For this review, take the finished solid that the model builds, in its own axes (mm). Face numbers are marked on the shaded views. A direction names the side the tool comes from. Coordinates: 2 decimals unless noted, no trailing zeros. Order: outer loops, then holes, each group sorted by start corner. A loop starts at its lowest first (then second) coordinate and runs counter-clockwise, first axis right, second up. Notation, with made-up numbers: (9, 85) - (14, 85) arc R25 cw to (14, 113) - close; hole circle Ø7 at (-1.5, 88.25). An arc over 180 degrees is marked (long way). One line per item, written item: value. Start each with the question number.
(1) Clearance check with flat-ended pins moving along their axes: pin 1 (2 mm diameter, centred on y = 21, z = 2.5, fed in from -X); pin 2 (2 mm diameter, centred on y = 14, z = 2, fed in from -X); pin 3 (1.6 mm diameter, centred on x = 34.5, z = 2.5, fed in from -Y). State where each tip first meets the part, or that it passes through.
(2) Consider section C-C on y = 10. Write out the cut boundary in (x, z), then the cut area to 3 significant figures.
(3) To check wall thickness, follow line 1 along X through (y, z) = (6.5, 3.7); line 2 along X through (y, z) = (4.25, 3.25); line 3 along Y through (x, z) = (44.5, 3.1). State the ranges of each line that lie inside material, in increasing order.
(4) Consider section D-D on y = 16.45. Write out the cut boundary in (x, z).
(5) Consider section A-A on x = 44.5. Write out the cut boundary in (y, z).
(6) For the marked faces 1, 2 and 3, list the 3-axis set-ups (+Z, -Z, +X, -X, +Y, -Y) from which the entire face can be reached by the end or side of a thin tool; tool diameter is ignored.
(7) Mouldability with a two-part tool opening along X and no side actions: class the marked faces 4, 5, 6 and 7 as released by +X, released by -X, zero draft, split by the parting line, or undercut.
(8) Consider section B-B on z = 0.75. Write out the cut boundary in (x, y), then the cut area to 3 significant figures.
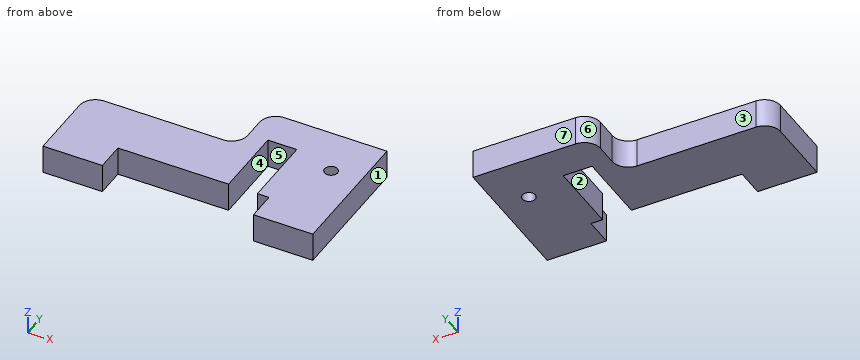
```python
from build123d import *

# Parameters (mm, degrees)
MODEL_R             = 1.2
BOSS_EXTRUDE1_DEPTH = 5.35


with BuildPart() as part:
    # Model → Boss-Extrude1 (new body)
    with BuildSketch(Plane.XY):
        with BuildLine():
            Line((39, 0), (50, 0))
            Line((50, 0), (50, 25.45))
            Line((50, 25.45), (31, 25.45))
            ThreePointArc((31, 25.45), (28.878679656, 24.571320344), (28, 22.45))
            Line((28, 22.45), (28, 18.45))
            ThreePointArc((28, 18.45), (27.121320344, 16.328679656), (25, 15.45))
            Line((25, 15.45), (3, 15.45))
            ThreePointArc((3, 15.45), (0.878679656, 14.571320344), (0, 12.45))
            Line((0, 12.45), (0, 0))
            Line((0, 0), (11, 0))
            Line((11, 0), (11, 5.35))
            Line((11, 5.35), (31.5, 5.35))
            Line((31.5, 5.35), (31.5, 18.85))
            Line((31.5, 18.85), (36.85, 18.85))
            Line((36.85, 18.85), (36.85, 5.35))
            Line((36.85, 5.35), (39, 5.35))
            Line((39, 5.35), (39, 0))
        make_face()
        with Locations((44.5, 16.45)):
            Circle(MODEL_R, mode=Mode.SUBTRACT)
    extrude(amount=BOSS_EXTRUDE1_DEPTH)


solid = part.part
```
Geometry check:
1. pin 1: stops at x = 28
1. pin 2: stops at x = 0.05
1. pin 3: stops at y = 18.85
2. outline: (0, 0) - (31.5, 0) - (31.5, 5.35) - (0, 5.35) - close; (36.85, 0) - (50, 0) - (50, 5.35) - (36.85, 5.35) - close
2. area: 239 mm^2
3. line 1: x = 0 to 31.5, 36.85 to 50
3. line 2: x = 0 to 11, 39 to 50
3. line 3: y = 0 to 15.25, 17.65 to 25.45
4. outline: (27.24, 0) - (31.5, 0) - (31.5, 5.35) - (27.24, 5.35) - close; (36.85, 0) - (43.3, 0) - (43.3, 5.35) - (36.85, 5.35) - close; (45.7, 0) - (50, 0) - (50, 5.35) - (45.7, 5.35) - close
5. outline: (0, 0) - (15.25, 0) - (15.25, 5.35) - (0, 5.35) - close; (17.65, 0) - (25.45, 0) - (25.45, 5.35) - (17.65, 5.35) - close
6. face 1: +Z, -Z, +X, +Y, -Y
6. face 2: +Z, -Z, -Y
6. face 3: +Z, -Z, -X, +Y
7. face 4: undercut
7. face 5: undercut
7. face 6: released by -X
7. face 7: zero draft
8. outline: (0, 0) - (11, 0) - (11, 5.35) - (31.5, 5.35) - (31.5, 18.85) - (36.85, 18.85) - (36.85, 5.35) - (39, 5.35) - (39, 0) - (50, 0) - (50, 25.45) - (31, 25.45) arc R3 ccw to (28, 22.45) - (28, 18.45) arc R3 cw to (25, 15.45) - (3, 15.45) arc R3 ccw to (0, 12.45) - close; hole circle Ø2.4 at (44.5, 16.45)
8. area: 764 mm^2
